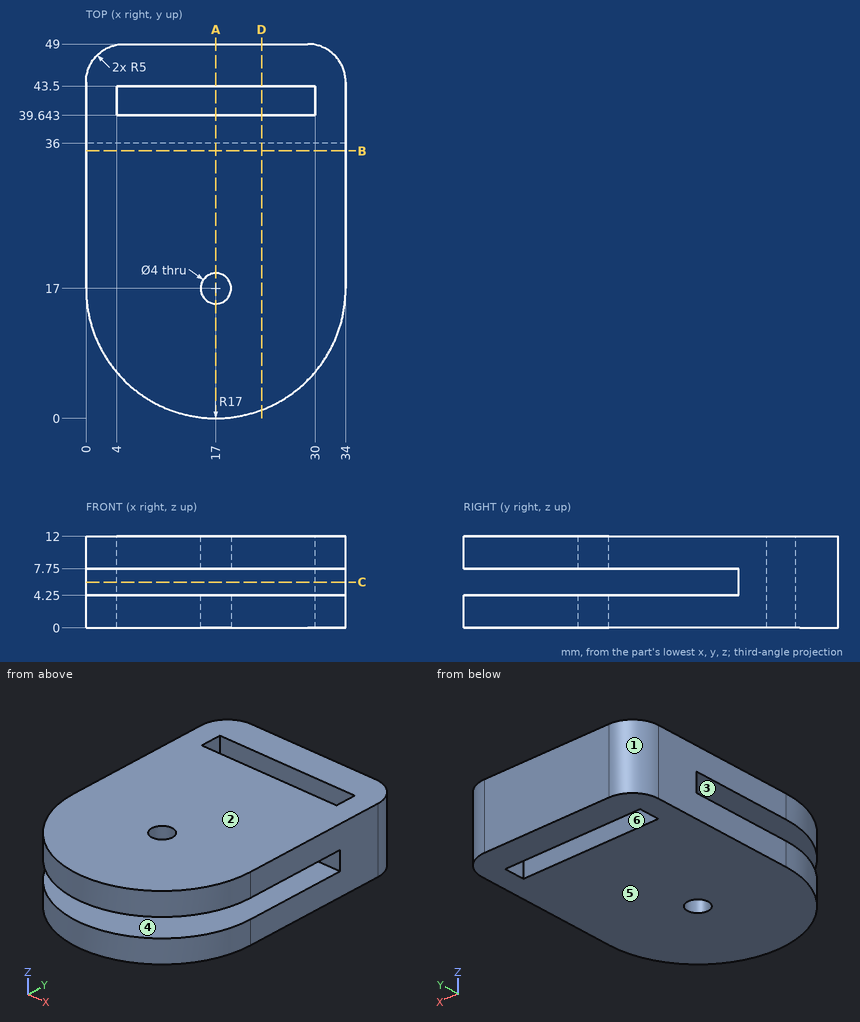
The figure shows three views and two pictorial views of one solid part (mm, origin at its lowest corner). Answer the questions. A direction names the side the tool comes from. Round coordinates to 2 decimals unless told otherwise and drop trailing zeros. Order: outer loops, then holes, each group sorted by start corner. A loop starts at its lowest first (then second) coordinate and runs counter-clockwise, first axis right, second up. Notation, with made-up numbers: M 49,-12.75 L 53,-12.75 A29 ccw 53,8.25 Z; hole C 12.25,83.5 d11. An arc over 180 degrees is marked long. Put each result on its own line as item: value. Start each with the question number.
Q1. Section B-B, the plane y = 35 is taken. Write down the section's boundary in (x, z).
Q2. Straight lines are drawn through the part: L1, parallel to Y at x = 17, z = 1.6; L2, parallel to Z at x = 3, y = 23.5; L3, parallel to Y at x = 5.5, z = 5.25. For each, find the intervals that lie inside material, in ascending order. Write a range as [from, to].
Q3. Section C-C, the plane z = 6 is taken. Write down the section's boundary in (x, y), and give its area (3 significant figures).
Q4. For a pull along Z with two mould halves and no side action, classify the marked faces 1, 2, 3 and 4 as pulls with the +Z half, pulls with the -Z half, needs draft (parallel to the pull), parting line crosses it, or undercut.
Q5. A tool of negligible diameter and unlimited length cuts with its end or side. For the marked faces 5 and 6, from which of +Z, -Z, +X, -X, +Y, -Y can it reach the whole face along a straight path? Write none if from no direction.
Q6. Flat-ended cylindrical pins translate along their axes: pin 1 (6 mm diameter, centred on y = 28.5, z = 2, fed in from -X); pin 2 (3 mm diameter, centred on x = 11.5, z = 5, fed in from -Y). Find the tip coordinate at first contact, or state that the pin passes through.
Q7. Section D-D, the plane x = 23 is taken. Write down the section's boundary in (y, z).
Q8. Section A-A, the plane x = 17 is taken. Write down the section's boundary in (y, z), and give its area (3 significant figures).
Findings below:
1. outline: M 0,0 L 34,0 L 34,4.25 L 0,4.25 Z; M 0,7.75 L 34,7.75 L 34,12 L 0,12 Z
2. L1: y = [0, 15], [19, 39.64], [43.5, 49]
2. L2: z = [0, 4.25], [7.75, 12]
2. L3: y = [36, 39.64], [43.5, 49]
3. outline: M 0,36 L 34,36 L 34,44 A5 ccw 29,49 L 5,49 A5 ccw 0,44 Z; hole M 4,39.64 L 30,39.64 L 30,43.5 L 4,43.5 Z
3. area: 331 mm^2
4. face 1: needs draft
4. face 2: pulls with the +Z half
4. face 3: undercut
4. face 4: undercut
5. face 5: -Z, +X, -X, +Y, -Y
5. face 6: +Z, -Z
6. pin 1: stops at x = 0
6. pin 2: stops at y = 0.53
7. outline: M 1.09,0 L 39.64,0 L 39.64,12 L 1.09,12 L 1.09,7.75 L 36,7.75 L 36,4.25 L 1.09,4.25 Z; M 43.5,0 L 49,0 L 49,12 L 43.5,12 Z
8. outline: M 0,0 L 15,0 L 15,4.25 L 0,4.25 Z; M 0,7.75 L 15,7.75 L 15,12 L 0,12 Z; M 19,0 L 39.64,0 L 39.64,12 L 19,12 L 19,7.75 L 36,7.75 L 36,4.25 L 19,4.25 Z; M 43.5,0 L 49,0 L 49,12 L 43.5,12 Z
8. area: 382 mm^2
